Verification items for the finished model (mm, model axes). Face numbers are marked on the shaded views. Round coordinates to 2 decimals unless told otherwise and drop trailing zeros. Order: outer loops, then holes, each group sorted by start corner. A loop starts at its lowest first (then second) coordinate and runs counter-clockwise, first axis right, second up. Notation, with made-up numbers: (-13, -39.5) -> (21, -39.5) arc R22 cw to (21, -33.5) -> close; hole circle Ø10 at (-9, -11.75). An arc over 180 degrees is marked (long way). Write item = value, one per line. Start each with the question number.
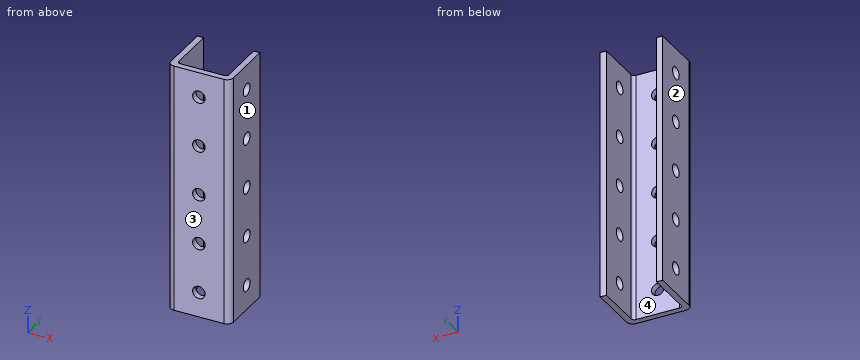
Autodesk Inventor part; units mm, degrees
ref_plane "YZ Plane" through (0, 0, 0) normal (1, 0, 0) x (0, 1, 0)
ref_plane "XZ Plane" through (0, 0, 0) normal (0, 1, 0) x (-1, 0, 0)
ref_plane "XY Plane" through (0, 0, 0) normal (0, 0, 1) x (1, 0, 0)
sketch "Sketch1" plane through (0, 0, 0) normal (0, 0, 1) x (1, 0, 0)
  line L0 (3.175, 0) -> (28.575, 0)
  line L1 (31.75, 3.175) -> (31.75, 28.575)
  line L2 (0, 28.575) -> (0, 3.175)
  line L3 (4.7625, 3.175) -> (26.9875, 3.175)
  line L4 (28.575, 4.7625) -> (28.575, 28.575)
  line L5 (3.175, 28.575) -> (3.175, 4.7625)
  line L6 (0, 28.575) -> (3.175, 28.575)
  line L7 (28.575, 28.575) -> (31.75, 28.575)
  arc A0 (3.175, 4.7625) -> (4.7625, 3.175) centre (4.7625, 4.7625) ccw
  arc A1 (26.9875, 3.175) -> (28.575, 4.7625) centre (26.9875, 4.7625) ccw
  arc A2 (0, 3.175) -> (3.175, 0) centre (3.175, 3.175) ccw
  arc A3 (28.575, 0) -> (31.75, 3.175) centre (28.575, 3.175) ccw
  point P0 (0, 0)
  point P1 (0, 0)
  point P2 (31.75, 0)
  dimension "d0" = 31.75
  dimension "d1" = 28.575
  dimension "d2" = 1.5875
  dimension "d3" = 3.175
extrude "Extrusion1" add sketch "Sketch1" along normal blind 127
sketch "Sketch2" plane through (31.75, 3.175, 0) normal (1, 0, 0) x (0, 0, -1)
  line L0 (-127, 0) -> (-127, 25.4)
  line L1 (0, 0) -> (-127, 0)
  line L2 (-127, 12.7) -> (-114.3, 12.7)
  point P0 (0, -3.175)
  dimension "d6" = 12.7
sketch "Sketch3" plane through (3.175, 0, 0) normal (0, -1, 0) x (1, 0, 0)
  line L0 (0, 127) -> (25.4, 127)
  line L1 (0, 0) -> (0, 127)
  line L2 (12.7, 127) -> (12.7, 114.3)
  point P0 (-3.175, 0)
  dimension "d7" = 12.7
hole "Hole1" at (31.75, 15.875, 114.3) direction (-1, 0, 0) diameter 6.35 end through all
hole "Hole2" at (15.875, 0, 114.3) direction (0, 1, 0) diameter 6.35 end through all
pattern_linear "Rectangular Pattern1" count 5 spacing 25.4 along (0, 0, -1) of "Hole1", "Hole2"
properties part number "5 in bar"
(1) Depth check by flat-ended pin: pin 1 (11 mm diameter, centred on x = 15.5, z = 65.5, fed in from +Y) (3 decimals); pin 2 (7.5 mm diameter, centred on y = 15.875, z = 88.9, fed in from -X). Enter the tip coordinate at first touch or a pass-through.
(2) Cross-section at C-C (x = 9). Enter the section's corners in (y, z) (3 decimals).
(3) Draft check along X on the marked faces 1, 2, 3 and 4. Enter one of: +X half, -X half, draft (parallel to the pull), parting line (faces both ways), or undercut.
(4) Cross-section at B-B (z = 88.9). Give the number of separate pieces and of enclosed holes in the cut face, and give its area (3 significant figures).
(5) Cross-section at A-A (y = 10.5). Enter the section's corners in (x, z) (3 decimals), and give its area (3 significant figures).
(6) Scan lines: line 1 along Z through (x, y) = (3, 16); line 2 along X through (y, z) = (24.75, 113) (3 decimals); line 3 along Y through (x, z) = (27, 93.5). Record each from-to range of solid material in increasing order. Write a range as from..to.
Outcome:
q1.pin_1 = 3.175
q1.pin_2 = 0
q2.outline = (0, 0) -> (3.175, 0) -> (3.175, 127) -> (0, 127) -> close
q3.face_1 = +X half
q3.face_2 = -X half
q3.face_3 = draft
q3.face_4 = undercut
q4.separate_pieces = 4
q4.enclosed_holes = 0
q4.area = 198 mm^2
q5.outline = (0, 0) -> (3.175, 0) -> (3.175, 127) -> (0, 127) -> close; (28.575, 0) -> (31.75, 0) -> (31.75, 127) -> (28.575, 127) -> close
q5.area = 806 mm^2
q6.line_1 = 0..9.53, 15.87..34.93, 41.27..60.33, 66.67..85.73, 92.07..111.13, 117.47..127
q6.line_2 = 0..3.175, 28.575..31.75
q6.line_3 = 0..3.18
